Geometry: final body of the model. Coordinates: model frame, mm. Face numbers are marked on the shaded views. A direction names the side the tool comes from. Coordinates: 2 decimals unless noted, no trailing zeros. Loops run counter-clockwise (first coordinate to the right, second up) from the corner with the lowest first, then second, coordinate; pieces in that order, holes last. Notation, with made-up numbers: (-34, 70.25) - (17, 70.25) arc R31 ccw to (17, 104.25) - close; hole circle Ø10 at (-14, 82). An arc over 180 degrees is marked (long way). Answer in a Markdown table with one row per item.
from build123d import *

# Parameters (mm, degrees)
SKETCH012_R     = 4
PAD005_DEPTH    = 3
PAD006_DEPTH    = 56
POCKET007_DEPTH = 20
SKETCH016_R     = 7
POCKET008_DEPTH = 3
SKETCH018_R     = 2.1
POCKET010_DEPTH = 3
SKETCH019_R     = 5
PAD007_DEPTH    = 3
SKETCH020_R     = 1.5
PAD008_DEPTH    = 4.5
PAD009_DEPTH    = 10
FILLET_R        = 9
FILLET001_R     = 6


with BuildPart() as part:
    # Sketch012 → Pad005 (new body)
    with BuildSketch(Plane.YZ):
        with BuildLine():
            Line((-13.6486038997, -19.3575724611), (-19.5095708271, -33.1651452629))
            Line((-19.5095708271, -33.1651452629), (-74.0996091673, -39.8679591502))
            ThreePointArc((-74.0996091673, -39.8679591502), (-78.4529932085, -45.4400366254), (-72.8809157334, -49.7934206666))
            Line((-72.8809157334, -49.7934206666), (-18.2908773931, -43.0906067793))
            ThreePointArc((-18.2908773931, -43.0906067793), (-13.4914205956, -41.1515003634), (-10.3045222925, -37.0724565478))
            Line((-10.3045222925, -37.0724565478), (-4.4435553652, -23.264883746))
            ThreePointArc((6.6243568489, -6.092445842), (0.3541186357, -14.2041191435), (-4.4435553652, -23.264883746))
            ThreePointArc((6.6243568489, -6.092445842), (3.5165801564, 8.2845436811), (-8.9842037096, 0.5329950324))
            ThreePointArc((-13.6486038997, -19.3575724611), (-10.4635797031, -9.6122786293), (-8.9842037096, 0.5329950324))
        make_face()
        Circle(SKETCH012_R, mode=Mode.SUBTRACT)
    extrude(amount=PAD005_DEPTH)

    # Sketch013 (on Face11 of Pad005) → Pad006 (join)
    with BuildSketch(Plane(origin=(0, 0, 0), x_dir=(0, 1, 0), z_dir=(-1, 0, 0))):
        Polygon((-111.7906110668, 61.1197443885), (-48.2676573618, 53.3201064106), (-51.0706522601, 30.4915449228), (-114.5936059651, 38.2911829007), align=None)
    extrude(amount=PAD006_DEPTH)

    # Sketch015 (on Face15 of Pad006) → Pocket007 (cut)
    with BuildSketch(Plane(origin=(0, 5.7327727551, -46.6896873101), x_dir=(0, 0.9925461516, 0.1218693434), z_dir=(0, 0.1218693434, -0.9925461516))):
        Polygon((-115.4059639217, -3), (-57.4059639217, -3), (-57.4059639217, -10), (-66.4059639217, -10), (-66.4059639217, -13), (-57.4059639217, -13), (-57.4059639217, -53), (-115.4059639217, -53), (-115.4059639217, -13), (-107.6059639217, -13), (-107.6059639217, -10), (-115.4059639217, -10), align=None)
    extrude(amount=-POCKET007_DEPTH, mode=Mode.SUBTRACT)

    # Sketch016 (on Face14 of Pocket007) → Pocket008 (cut)
    with BuildSketch(Plane.YZ):
        with Locations((-92.1658353164, -48.6350266606)):
            Circle(SKETCH016_R)
    extrude(amount=-POCKET008_DEPTH, mode=Mode.SUBTRACT)

    # Sketch018 → Pocket010 (cut)
    with BuildSketch(Plane(origin=(-13, 0, 0), x_dir=(0, 1, 0), z_dir=(-1, 0, 0))):
        with Locations((-57.4788589785, 39.8422072873)):
            Circle(SKETCH018_R)
        with Locations((-56.3820348878, 48.7751226521)):
            Circle(SKETCH018_R)
        with Locations((-107.403930406, 45.9722352606)):
            Circle(SKETCH018_R)
        with Locations((-106.3071063154, 54.9051506254)):
            Circle(SKETCH018_R)
    extrude(amount=-POCKET010_DEPTH, mode=Mode.SUBTRACT)

    # Sketch019 → Pad007 (join)
    with BuildSketch(Plane(origin=(-56, 0, 0), x_dir=(0, 1, 0), z_dir=(-1, 0, 0))):
        with BuildLine():
            ThreePointArc((-8.9842037096, -0.5329950324), (3.5165801564, -8.2845436811), (6.6243568489, 6.092445842))
            ThreePointArc((-4.4435553652, 23.264883746), (0.3541186357, 14.2041191435), (6.6243568489, 6.092445842))
            Line((-4.4435553652, 23.264883746), (-10.3045222925, 37.0724565478))
            ThreePointArc((-10.3045222925, 37.0724565478), (-13.4914205956, 41.1515003634), (-18.290877393, 43.0906067793))
            Line((-18.290877393, 43.0906067793), (-72.8809157333, 49.7934206666))
            ThreePointArc((-72.8809157333, 49.7934206666), (-78.4529932085, 45.4400366254), (-74.0996091673, 39.8679591502))
            Line((-19.5095708271, 33.1651452629), (-74.0996091673, 39.8679591502))
            Line((-13.6486038997, 19.3575724611), (-19.5095708271, 33.1651452629))
            ThreePointArc((-8.9842037096, -0.5329950324), (-10.4635797031, 9.6122786293), (-13.6486038997, 19.3575724611))
        make_face()
        Circle(SKETCH019_R, mode=Mode.SUBTRACT)
    extrude(amount=PAD007_DEPTH)

    # Sketch020 (on Face17 of Pad007) → Pad008 (join)
    with BuildSketch(Plane(origin=(-56, 0, 0), x_dir=(0, 1, 0), z_dir=(-1, 0, 0))):
        with Locations((-92.1658353164, 48.6350266606)):
            Circle(SKETCH020_R)
    extrude(amount=PAD008_DEPTH)

    # Sketch021 (on Face9 of Pad008) → Pad009 (join)
    with BuildSketch(Plane(origin=(0, 4.9406220229, -40.2381373244), x_dir=(0, 0.9925461516, 0.1218693434), z_dir=(0, 0.1218693434, -0.9925461516))):
        with BuildLine():
            Line((-27.4059639217, 0), (-54.4059639217, 0))
            Line((-54.4059639217, 0), (-54.4059639217, -17))
            ThreePointArc((-27.4059639217, 0), (-42.2983611114, -6.2885456399), (-54.4059639217, -17))
        make_face()
        with BuildLine():
            Line((-54.4059639217, -39), (-54.4059639217, -56))
            Line((-27.4059639217, -56), (-54.4059639217, -56))
            ThreePointArc((-54.4059639217, -39), (-42.2983611114, -49.7114543601), (-27.4059639217, -56))
        make_face()
    extrude(amount=-PAD009_DEPTH)

    # Fillet
    fillet_edges = [part.edges().sort_by_distance(p)[0] for p in [
        (0, -113.192109, -49.705464),
        (-56, -113.192109, -49.705464),
    ]]
    fillet(fillet_edges, radius=FILLET_R)

    # Fillet001
    fillet001_edges = [part.edges().sort_by_distance(p)[0] for p in [
        (-53, -110.031666, -50.828675),
        (-3, -110.031666, -50.828675),
    ]]
    fillet(fillet001_edges, radius=FILLET001_R)


with BuildPart() as part_1:
    # Body004 placement: moved
    add(part.part.moved(Location((28, 16.5, -26.5))))


solid = part_1.part
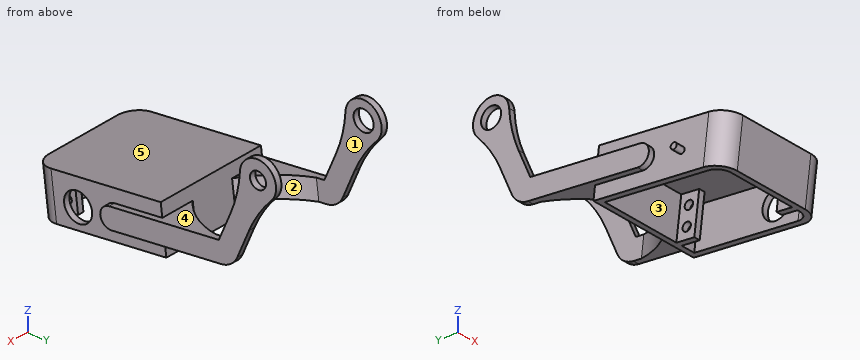
(1) First-contact query: pin 1 Ø12 at (x, y) = (16, -61) entering from -Z; pin 2 Ø5 at (y, z) = (-19, -60.5) entering from -X; pin 3 Ø10 at (x, z) = (-19.5, -48.5) entering from -Y; pin 4 Ø3 at (x, y) = (19, -65) entering from +Z. Flat tips, straight axial feed; report the tip coordinate or a pass-through.
Verdict:
| item | result |
|---|---|
| pin 1 | stops at z = -64 |
| pin 2 | stops at x = -31 |
| pin 3 | passes through |
| pin 4 | stops at z = -60.54 |
(2) Pull-direction query (Y, two-part tool) for the marked faces 1, 2 and 3; classes: pulls with the +Y half, pulls with the -Y half, needs draft (parallel to the pull), parting line crosses it, or undercut.
Verdict:
| item | result |
|---|---|
| face 1 | needs draft |
| face 2 | pulls with the +Y half |
| face 3 | undercut |
(3) Ray query, probe 1 along X at (y, z) = (-86, -73.5); probe 2 along Z at (x, y) = (-29.6, 16.5); probe 3 along X at (y, z) = (-12.5, -68). Return the intervals inside material, ascending.
Verdict:
| item | result |
|---|---|
| probe 1 | x = -28 to -25, 25 to 28 |
| probe 2 | z = -41.26 to -31.5, -21.5 to -17.5 |
| probe 3 | x = -31 to -25.98, 25.98 to 31 |
(4) Cut plane C-C on x = -8.5. Output: boundary loops of the cut face in (y, z), then the cut area to 3 significant figures.
Verdict:
| item | result |
|---|---|
| outline | (-98.09, -64.79) - (-95.29, -87.62) - (-92.31, -87.25) - (-94.75, -67.4) - (-37.18, -60.33) - (-34.75, -80.19) - (-31.77, -79.82) - (-34.57, -56.99) - close |
| area | 312 mm² |
(5) Cut plane D-D on y = -53. Output: boundary loops of the cut face in (x, z).
Verdict:
| item | result |
|---|---|
| outline | (-31, -75.88) - (-28, -75.88) - (-28, -82.43) - (-25, -82.43) - (-25, -62.28) - (25, -62.28) - (25, -82.43) - (28, -82.43) - (28, -75.88) - (31, -75.88) - (31, -65.8) - (28, -65.8) - (28, -59.25) - (-28, -59.25) - (-28, -65.8) - (-31, -65.8) - close |
(6) Cut plane B-B on y = 16.5. Output: boundary loops of the cut face in (x, z), then the cut area to 3 significant figures.
Verdict:
| item | result |
|---|---|
| outline | (-31, -41.26) - (-28, -41.26) - (-28, -31.5) - (-31, -31.5) - close; (-31, -21.5) - (-28, -21.5) - (-28, -17.5) - (-31, -17.5) - close; (28, -41.26) - (31, -41.26) - (31, -30.5) - (28, -30.5) - close; (28, -22.5) - (31, -22.5) - (31, -17.5) - (28, -17.5) - close |
| area | 88.6 mm² |
(7) Access query for the marked faces 4 and 5. Directions: +Z, -Z, +X, -X, +Y, -Y. A direction counts if a zero-diameter tool reaches every point of the face in a straight line with its end or side. Return the directions, or none.
Verdict:
| item | result |
|---|---|
| face 4 | +Z, +X |
| face 5 | +Z, +X, -X, -Y |
(8) Cut plane A-A on z = -34.5. Output: boundary loops of the cut face in (x, y).
Verdict:
| item | result |
|---|---|
| outline | (-31, 6.39) - (-28, 6.39) - (-28, 21.44) - (-31, 21.44) - close; (28, 6.39) - (31, 6.39) - (31, 21.44) - (28, 21.44) - close |
